Input: dimensioned drawing with shaded views. Units: mm. Origin: part minimum x, y, z. Round coordinates to 2 decimals unless told otherwise and drop trailing zeros. Loops run counter-clockwise (first coordinate to the right, second up) from the corner with the lowest first, then second, coordinate; pieces in that order, holes last.
Item 1: Section query D-D on x = 28.5. Return loops of the section in (y, z).
Item 2: Section query C-C on y = 3.5. Return loops of the section in (x, z).
Item 3: Section query B-B on z = 5.5. Return loops of the section in (x, y).
Item 4: Ray query, L1, parallel to X at y = 4.1, z = 6; L2, parallel to X at y = 0.85, z = 6; L3, parallel to Y at x = 37, z = 2. Return the intervals inside material, ascending.
Item 5: Section query A-A on x = 12. Return loops of the section in (y, z).
Item 6: Pull-direction query (Y, two-part tool) for the marked faces 1, 2 and 3; classes: released by +Y, released by -Y, zero draft, split by the parting line, or undercut.
Item 7: First-contact query: P1, Ø3.5, axis at x = 12, z = 6, coming from the +Y side; P2, Ø1, axis at x = 89.5, y = 1.5, coming from the -Z side. Flat tips, straight axial feed; report the tip coordinate or a pass-through.
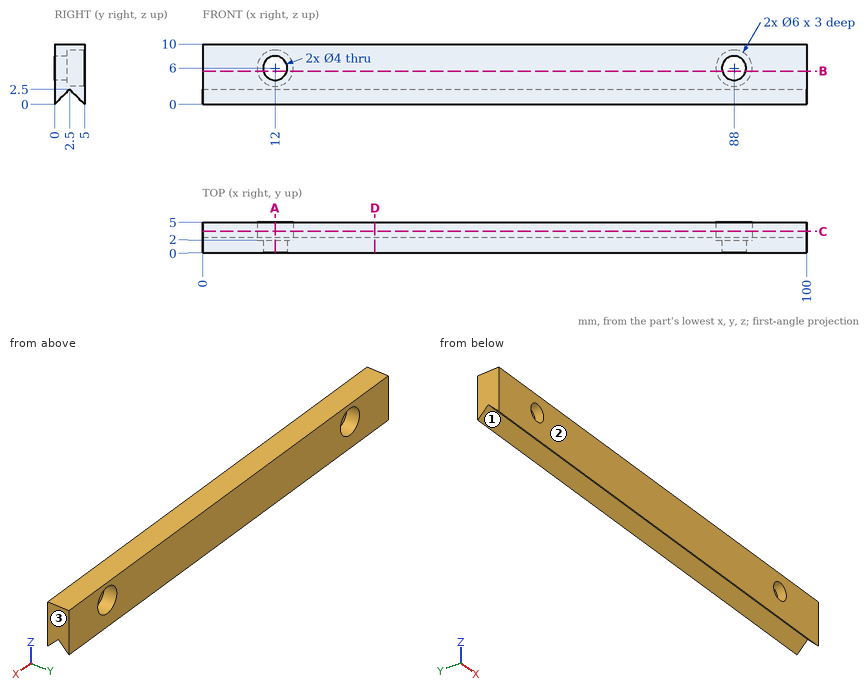
Data:
1. outline: (0, 0) - (2.5, 2.5) - (5, 0) - (5, 10) - (0, 10) - close
2. outline: (0, 1.5) - (100, 1.5) - (100, 10) - (0, 10) - close; hole circle Ø6 at (12, 6); hole circle Ø6 at (88, 6)
3. outline: (0, 0) - (10.06, 0) - (10.06, 2) - (9.04, 2) - (9.04, 5) - (0, 5) - close; (13.94, 0) - (86.06, 0) - (86.06, 2) - (85.04, 2) - (85.04, 5) - (14.96, 5) - (14.96, 2) - (13.94, 2) - close; (89.94, 0) - (100, 0) - (100, 5) - (90.96, 5) - (90.96, 2) - (89.94, 2) - close
4. L1: x = 0 to 9, 15 to 85, 91 to 100
4. L2: x = 0 to 10, 14 to 86, 90 to 100
4. L3: y = 0 to 2, 3 to 5
5. outline: (0, 0) - (2.5, 2.5) - (5, 0) - (5, 3) - (2, 3) - (2, 4) - (0, 4) - close; (0, 8) - (2, 8) - (2, 9) - (5, 9) - (5, 10) - (0, 10) - close
6. face 1: undercut
6. face 2: released by -Y
6. face 3: zero draft
7. P1: passes through
7. P2: stops at z = 1
